Input: part model. Units: mm. Frame: model coordinates. Face numbers are marked on the shaded views. A direction names the side the tool comes from. Coordinates: 2 decimals unless noted, no trailing zeros. Order: outer loops, then holes, each group sorted by start corner. A loop starts at its lowest first (then second) coordinate and runs counter-clockwise, first axis right, second up. Notation, with made-up numbers: (43, 50) - (79, 50) arc R16 cw to (79, 74) - close; hole circle Ø1 at (81, -21.75). An arc over 180 degrees is marked (long way). One line per question, with ' | ' between items.
from build123d import *

# Parameters (mm, degrees)
BOSS_EXTRUDE1_DEPTH = 40
SKETCH3_R           = 3.5
CUT_EXTRUDE1_DEPTH  = 32
SKETCH2_R           = 8
CUT_EXTRUDE2_DEPTH  = 32
CUT_EXTRUDE3_DEPTH  = 6
BOSS_EXTRUDE3_DEPTH = 4
FILLET1_R           = 4
FILLET4_R           = 2


with BuildPart() as part:
    # Sketch1 → Boss-Extrude1 (new body)
    with BuildSketch(Plane.XY):
        Polygon((0, 0), (0, 40), (-30, 40), (-30, 44), (6, 44), (6, 12), (26, 12), (26, 0), align=None)
    extrude(amount=BOSS_EXTRUDE1_DEPTH)

    # Sketch3 → Cut-Extrude1 (cut)
    with BuildSketch(Plane(origin=(0, 12, 0), x_dir=(1, 0, 0), z_dir=(0, 1, 0))):
        with Locations(Location((16, -20, 0), (0, 0, 270))):
            Circle(SKETCH3_R)
    extrude(amount=-CUT_EXTRUDE1_DEPTH, mode=Mode.SUBTRACT)

    # Sketch2 → Cut-Extrude2 (cut)
    with BuildSketch(Plane(origin=(0, 44, 0), x_dir=(1, 0, 0), z_dir=(0, 1, 0))):
        with Locations(Location((-14, -24, 0), (0, 0, 270))):
            Circle(SKETCH2_R)
    extrude(amount=-CUT_EXTRUDE2_DEPTH, mode=Mode.SUBTRACT)

    # Sketch4 → Cut-Extrude3 (cut)
    with BuildSketch(Plane(origin=(0, 12, 0), x_dir=(1, 0, 0), z_dir=(0, 1, 0))):
        Polygon((16, -26.639528096), (21.75, -23.319764048), (21.75, -16.680235952), (16, -13.360471904), (10.25, -16.680235952), (10.25, -23.319764048), align=None)
    extrude(amount=-CUT_EXTRUDE3_DEPTH, mode=Mode.SUBTRACT)

    # Sketch5 → Boss-Extrude3 (add)
    with BuildSketch(Plane(origin=(0, 0, 0), x_dir=(-1, 0, 0), z_dir=(0, 0, -1))):
        Polygon((-26, 12), (-6, 32), (-6, 12), align=None)
        Polygon((0, 10), (0, 40), (30, 40), align=None)
    extrude(amount=-BOSS_EXTRUDE3_DEPTH)

    # Fillet1
    fillet1_edges = [part.edges().sort_by_distance(p)[0] for p in [
        (26, 6, 0),
        (-30, 42, 40),
        (26, 6, 40),
        (-30, 42, 0),
    ]]
    fillet(fillet1_edges, radius=FILLET1_R)

    # Fillet4
    fillet4_edges = [part.edges().sort_by_distance(p)[0] for p in [
        (11, 0, 0),
        (0, 0, 20),
        (6, 44, 20),
        (6, 28, 40),
        (-10, 44, 40),
        (0, 20, 40),
        (11, 0, 40),
        (6, 38, 0),
        (26, 0, 20),
        (24.828427125, 0, 1.171572875),
        (24.828427125, 0, 38.828427125),
        (-30, 44, 20),
        (-28.828427125, 44, 1.171572875),
        (-28.828427125, 44, 38.828427125),
        (-10, 44, 0),
    ]]
    fillet(fillet4_edges, radius=FILLET4_R)


solid = part.part
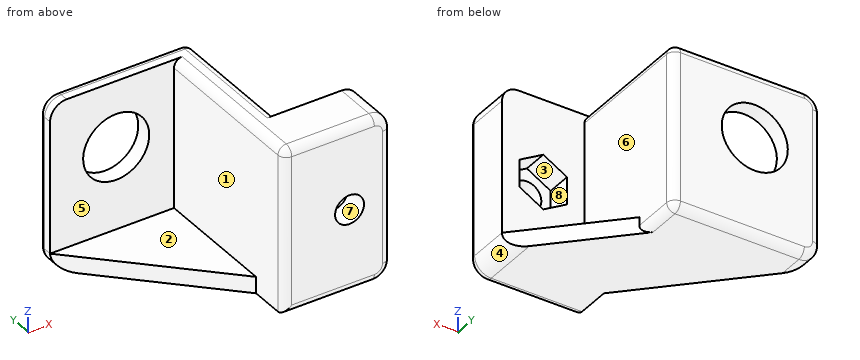
Item 1: Draft query along Z for the marked faces 1, 2, 3 and 4. Return one class per face: released by +Z, released by -Z, zero draft, split by the parting line, or undercut.
Data:
face 1: zero draft | face 2: released by +Z | face 3: undercut | face 4: released by -Z
Item 2: Section C-C on z = 21. Return the cut outline in (x, y).
Data:
outline: (-30, 40) - (-21.42, 40) - (-21.42, 44) - (-28, 44) arc R2 ccw to (-30, 42) - close; (-6.58, 40) - (0, 40) - (0, 2) arc R2 ccw to (2, 0) - (12.65, 0) - (12.65, 6) - (10.25, 6) - (10.25, 12) - (6, 12) - (6, 42) arc R2 ccw to (4, 44) - (-6.58, 44) - close; (19.35, 0) - (24, 0) arc R2 ccw to (26, 2) - (26, 12) - (21.75, 12) - (21.75, 6) - (19.35, 6) - close
Item 3: Access query for the marked faces 5, 6, 7 and 8. Directions: +Z, -Z, +X, -X, +Y, -Y. A direction counts if a zero-diameter tool reaches every point of the face in a straight line with its end or side. Return the directions, or none.
Data:
face 5: +Z, -X, -Y | face 6: +Z, +X, +Y | face 7: +Y, -Y | face 8: +Y
Item 4: Section D-D on z = 25. Return the cut outline in (x, y), and give its area (3 significant figures).
Data:
outline: (-30, 40) - (-21.94, 40) - (-21.94, 44) - (-28, 44) arc R2 ccw to (-30, 42) - close; (-6.06, 40) - (0, 40) - (0, 2) arc R2 ccw to (2, 0) - (24, 0) arc R2 ccw to (26, 2) - (26, 12) - (18.84, 12) - (18.84, 6) - (13.16, 6) - (13.16, 12) - (6, 12) - (6, 42) arc R2 ccw to (4, 44) - (-6.06, 44) - close | area: 523 mm^2
Item 5: Section A-A on y = 8.5. Return the cut outline in (x, z), and give its area (3 significant figures).
Data:
outline: (0, 0) - (22, 0) arc R4 ccw to (26, 4) - (26, 36) arc R4 ccw to (22, 40) - (2, 40) arc R2 ccw to (0, 38) - close; hole (10.25, 16.68) - (16, 13.36) - (21.75, 16.68) - (21.75, 23.32) - (16, 26.64) - (10.25, 23.32) - close | area: 918 mm^2
Item 6: Section B-B on x = -14. Return the cut outline in (y, z), and give its area (3 significant figures).
Data:
outline: (24, 0) - (42, 0) arc R2 ccw to (44, 2) - (44, 16) - (40, 16) - (40, 4) - (24, 4) - close; (40, 32) - (44, 32) - (44, 38) arc R2 ccw to (42, 40) - (40, 40) - close | area: 158 mm^2
Item 7: Contact query for flat-ended pins moving along their axis: P1, Ø8, axis at x = 16, z = 20, coming from the +Y side; P2, Ø3, axis at x = -2, z = 13, coming from the -Y side; P3, Ø1.5, axis at y = 20.5, z = 9, coming from the +X side; P4, Ø14.5, axis at x = -14, z = 24, coming from the +Y side. Output: stop coordinate, or through.
Data:
P1: y = 6 | P2: y = 40 | P3: x = 6 | P4: through
Item 8: Ray query, line 1 (X direction, y = 3, z = 20); line 2 (Y direction, x = -7, z = 18.5); line 3 (Z direction, x = -2, y = 12.5). Return the intervals inside material, ascending.
Data:
line 1: 0 to 12.5, 19.5 to 26 | line 2: 40 to 44 | line 3: 0 to 4
